```python
from build123d import *

# Parameters (mm, degrees)
CHAMFER_1_SIZE      = 1.2
CUT_EXTRUDE_1_REACH = 22.41
SKETCH_2_W          = 6
SKETCH_2_H          = 10


with BuildPart() as part:
    # Эскиз1 → Повернуть1 (revolve)
    with BuildSketch(Plane.XY, mode=Mode.PRIVATE) as revolve_1_sk:
        Polygon((-11.85, 0), (-13.45, 0), (-13.45, 7.4), (-12.15, 7.4), (-12.15, 3.6), (-11.85, 3.6), align=None)
    revolve(revolve_1_sk.sketch.rotate(Axis((0, 0, 0), (0, 1, 0)), 270), axis=Axis((0, 0, 0), (0, 1, 0)))

    # Фаска1
    chamfer_1_edges = [part.edges().sort_by_distance(p)[0] for p in [
        (0, 0, 13.45),
    ]]
    chamfer(chamfer_1_edges, length=CHAMFER_1_SIZE)

    # Эскиз2 → Вырез-Вытянуть1 (cut, up to next)
    with BuildSketch(Plane(origin=(0, 7.4, 0), x_dir=(1, 0, 0), z_dir=(0, 1, 0)), mode=Mode.PRIVATE) as cut_extrude_1_sk1:
        with Locations((0, 12)):
            Rectangle(SKETCH_2_W, SKETCH_2_H)
    cut_extrude_1_tool1 = extrude(cut_extrude_1_sk1.sketch, amount=-CUT_EXTRUDE_1_REACH, mode=Mode.PRIVATE) & part.part
    add(cut_extrude_1_tool1.solids().sort_by_distance((0, 7.4, -12))[0], mode=Mode.SUBTRACT)


solid = part.part
```
Read the model definition and answer for the solid it produces. Units are mm, in the model's axes. A direction names the side the tool comes from. Coordinates: 2 decimals unless noted, no trailing zeros. Write each loop counter-clockwise with the first axis right and the second up, starting at its lowest first coordinate (ties: lowest second). Pieces come first, ordered by that corner, then holes. Notation, with made-up numbers: (-24, 44.5) -> (-9, 44.5) arc R13 ccw to (-9, 56.5) -> close; hole circle Ø7 at (52.5, 44.5). An arc over 180 degrees is marked (long way). Answer as a JSON object with one key per item and string values.
Q1. A tool of negligible diameter and unlimited length cuts with its end or side. For faces 5 (the flat face through (3, 7.4, 12)), 6 (the flat face through (3, 4, -12)), from which of +Z, -Z, +X, -X, +Y, -Y can it reach the whole face along a straight path? Write none if from no direction.
The answers:
{"face 5": "+Z, -Z, +X, -X, +Y", "face 6": "-Z, +Y, -Y"}
Q2. The part is cut by section D-D on y = 2.5. Give the vertices of the cut face in (x, z), then the cut area to 3 significant figures.
The answers:
{"outline": "(-3, -13.11) -> (-3, -11.46) arc R11.85 cw (long way) to (3, -11.46) -> (3, -13.11) arc R13.45 ccw (long way) to start", "area": "117 mm2"}
Q3. Consider line 1 (X direction, y = 2.6, z = 0); line 2 (X direction, y = 5.35, z = 0); line 3 (Z direction, x = -0.25, y = 3). Determine where each line is inside the solid, lowest interval first. Write a range as [from, to].
The answers:
{"line 1": "x = [-13.45, -11.85], [11.85, 13.45]", "line 2": "x = [-13.45, -12.15], [12.15, 13.45]", "line 3": "z = [11.85, 13.45]"}
Q4. The part is cut by section C-C on y = 5.25. Give the vertices of the cut face in (x, z).
The answers:
{"outline": "(-3, -13.11) -> (-3, -11.77) arc R12.15 cw (long way) to (3, -11.77) -> (3, -13.11) arc R13.45 ccw (long way) to start"}
Q5. The part is cut by section B-B on x = 0. Give the vertices of the cut face in (y, z).
The answers:
{"outline": "(0, 11.85) -> (3.6, 11.85) -> (3.6, 12.15) -> (7.4, 12.15) -> (7.4, 13.45) -> (1.2, 13.45) -> (0, 12.25) -> close"}
Q6. The part is cut by section A-A on z = 0. Give the vertices of the cut face in (x, y), then the cut area to 3 significant figures.
The answers:
{"outline": "(-13.45, 1.2) -> (-12.25, 0) -> (-11.85, 0) -> (-11.85, 3.6) -> (-12.15, 3.6) -> (-12.15, 7.4) -> (-13.45, 7.4) -> close; (11.85, 0) -> (12.25, 0) -> (13.45, 1.2) -> (13.45, 7.4) -> (12.15, 7.4) -> (12.15, 3.6) -> (11.85, 3.6) -> close", "area": "20.0 mm2"}
Q7. Flat-ended cylindrical pins translate along their axes: pin 1 Ø1 at (x, y) = (-9, 4) entering from -Z; pin 2 Ø8 at (x, z) = (-9, 1) entering from -Y; pin 3 Ø1.8 at (y, z) = (3, -12.5) entering from -X; pin 4 Ø1.8 at (y, z) = (4.5, -12) entering from +X. Find the tip coordinate at first contact, or state that the pin passes through.
The answers:
{"pin 1": "stops at z = -10.42", "pin 2": "stops at y = 0", "pin 3": "stops at x = -6.81", "pin 4": "stops at x = 7.6"}
Q8. Determine the mould class of faces 1 (the cylindrical face through (-0.49, 5.47, 12.14)), 2 (the cylindrical face through (-0.55, 4.34, 13.44)), 3 (the flat face through (-12, 0, 0)), 4 (the flat face through (-3, 4, -12)) for opening direction X: pulls with the +X half, pulls with the -X half, needs draft (parallel to the pull), parting line crosses it, or undercut.
The answers:
{"face 1": "undercut", "face 2": "parting line crosses it", "face 3": "needs draft", "face 4": "undercut"}
